Autodesk Inventor part; units mm, degrees
ref_plane "YZ Plane" through (0, 0, 0) normal (1, 0, 0) x (0, 1, 0)
ref_plane "XZ Plane" through (0, 0, 0) normal (0, 1, 0) x (-1, 0, 0)
ref_plane "XY Plane" through (0, 0, 0) normal (0, 0, 1) x (1, 0, 0)
sketch "Sketch1" plane through (0, 0, 0) normal (0, 0, 1) x (1, 0, 0)
  line L0 (-7.5032, 0) -> (7.5032, 0)
  line L1 (0, -7.5032) -> (0, 7.5032)
  circle A0 centre (0, 0) radius 5.3594
  circle A1 centre (0, 0) radius 3.175
  dimension "d0" = 6.35
  dimension "d1" = 10.7188
extrude "Base" add sketch "Sketch1" along normal mid plane 3.683 contours A1 L1 A0 L0 | L0 A0 L1 A1 | A1 L0 A0 L1 | L1 A0 L0 A1
sketch "Sketch2" plane through (0, 0, 1.8415) normal (0, 0, 1) x (1, 0, 0)
  circle A0 centre (0, 0) radius 5.3594
  circle A1 centre (0, 0) radius 4.7625
  dimension "d4" = 9.525
extrude "Flange Cutaway" cut sketch "Sketch2" against normal blind 3.175
sketch "Sketch3" plane through (0, 0, 1.8415) normal (0, 0, 1) x (1, 0, 0)
  circle A0 centre (0, 0) radius 3.175
  circle A1 centre (0, 0) radius 4.7625
  circle A2 centre (0, 0) radius 3.683
  circle A3 centre (0, 0) radius 4.2545
  dimension "d11" = 0.508
  dimension "d12" = 0.508
extrude "Cutaway" cut sketch "Sketch3" against normal blind 0.1984 contours A3
mirror "Mirror1" about plane through (0, 0, 0) normal (0, 0, 1) of "Cutaway"
properties part number "bearing_1.125OD" material "Steel"
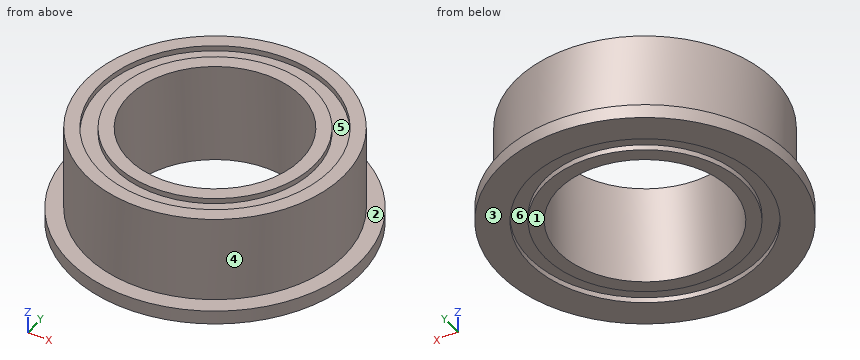
Input: part model. Units: mm. Frame: model coordinates. Face numbers are marked on the shaded views. A direction names the side the tool comes from. Give positions to 0.01 mm unless a question says otherwise; leave off trailing zeros. Loops run counter-clockwise (first coordinate to the right, second up) from the corner with the lowest first, then second, coordinate; pieces in that order, holes last. Notation, with made-up numbers: (82.5, 1) -> (89.5, 1) arc R16 ccw to (89.5, 31) -> close; hole circle Ø7 at (25.25, 1.25). An arc over 180 degrees is marked (long way). Answer as a JSON object with one key per item and string values. Group by question number.
Item 1: Reachability of the marked faces 1 and 2 from +Z, -Z, +X, -X, +Y, -Y: full face, straight path, thin tool, end or side. Return the list, or none.
Item 2: Pull-direction query (X, two-part tool) for the marked faces 3, 4, 5 and 6; classes: released by +X, released by -X, zero draft, split by the parting line, or undercut.
Item 3: Pin query (flat end, axial travel): P1, Ø1, axis at y = -3.5, z = 0.5, coming from the +X side; P2, Ø1.5, axis at x = 1.5, z = -0.5, coming from the -Y side; P3, Ø1, axis at y = -1, z = -0.5, coming from the +X side; P4, Ø2, axis at x = 1.5, y = -0.5, coming from the +Z side. Return the tip coordinate at first contact, or that it passes through.
Item 4: Line query: probe 1 along Y at (x, z) = (0, -1.7) (1 decimal); probe 2 along Y at (x, z) = (0, 0.9) (1 decimal); probe 3 along Y at (x, z) = (0.25, 1.7). Output: solid intervals per line, ascending.
Item 5: Cut plane D-D, the plane x = -4.5. Return the cut outline in (y, z), and give its area (3 significant figures).
Checks:
{
 "1": {"face 1": "-Z, +X, -X, +Y, -Y", "face 2": "+Z"},
 "2": {"face 3": "zero draft", "face 4": "split by the parting line", "face 5": "undercut", "face 6": "undercut"},
 "3": {"P1": "stops at x = 3.7", "P2": "stops at y = -4.7", "P3": "stops at x = 4.74", "P4": "passes through"},
 "4": {"probe 1": "y = -5.4 to -4.3, -3.7 to -3.2, 3.2 to 3.7, 4.3 to 5.4", "probe 2": "y = -4.8 to -3.2, 3.2 to 4.8", "probe 3": "y = -4.76 to -4.25, -3.67 to -3.17, 3.17 to 3.67, 4.25 to 4.76"},
 "5": {"outline": "(-2.91, -1.84) -> (2.91, -1.84) -> (2.91, -1.33) -> (1.56, -1.33) -> (1.56, 1.84) -> (-1.56, 1.84) -> (-1.56, -1.33) -> (-2.91, -1.33) -> close", "area": "12.9 mm²"}
}
